Part model, mm, in its own coordinate system. A direction names the side the tool comes from. Round coordinates to 2 decimals unless told otherwise and drop trailing zeros. Loops run counter-clockwise (first coordinate to the right, second up) from the corner with the lowest first, then second, coordinate; pieces in that order, holes last. Notation, with made-up numbers: (37, -0.5) -> (77, -0.5) arc R24 ccw to (77, 11.5) -> close; hole circle Ø8 at (42.25, 15). An arc over 180 degrees is marked (long way). Answer as a JSON object with one key per item and string values. Group by question number.
from build123d import *

# Parameters (mm, degrees)
EXTRUDE_1_DEPTH             = 10.5
FILLET_1_R                  = 0.3
FILLET_2_R                  = 2
HOLE_WIZARD_M52_D           = 4.2
HOLE_WIZARD_M52_CSINK_D     = 5.05
HOLE_WIZARD_M52_CSINK_ANGLE = 90


with BuildPart() as part:
    # Эскиз1 → Бобышка-Вытянуть1 (new body, symmetric)
    with BuildSketch(Plane.XY):
        with BuildLine():
            Line((-4, 0), (4, 0))
            Line((4, 0), (4, -0.8))
            Line((4, -0.8), (6.5, -0.8))
            Line((6.5, -0.8), (6.5, -1.6))
            ThreePointArc((6.5, -1.6), (4.386776199, -4.87777644), (1.5, -7.5))
            Line((1.5, -7.5), (-1.5, -7.5))
            ThreePointArc((-1.5, -7.5), (-4.386776199, -4.87777644), (-6.5, -1.6))
            Line((-6.5, -1.6), (-6.5, -0.8))
            Line((-6.5, -0.8), (-4, -0.8))
            Line((-4, -0.8), (-4, 0))
        make_face()
    extrude(amount=EXTRUDE_1_DEPTH, both=True)

    # Скругление1
    fillet_1_edges = [part.edges().sort_by_distance(p)[0] for p in [
        (6.5, -0.8, 0),
        (6.5, -1.6, 0),
        (-6.5, -1.6, 0),
        (-6.5, -0.8, 0),
        (-4, 0, 0),
        (4, 0, 0),
    ]]
    fillet(fillet_1_edges, radius=FILLET_1_R)

    # Скругление2
    fillet_2_edges = [part.edges().sort_by_distance(p)[0] for p in [
        (1.5, -7.5, 0),
        (-1.5, -7.5, 0),
    ]]
    fillet(fillet_2_edges, radius=FILLET_2_R)

    # Отверстие обработанное метчиком M52 (through all)
    with Locations(Plane(origin=(0, 0, 0), x_dir=(1, 0, 0), z_dir=(0, 1, 0))):
        with Locations((0, -4.5)):
            CounterSinkHole(HOLE_WIZARD_M52_D / 2, HOLE_WIZARD_M52_CSINK_D / 2, counter_sink_angle=HOLE_WIZARD_M52_CSINK_ANGLE)

    # Эскиз5 → Повернуть1 (revolve)
    with BuildSketch(Plane(origin=(0, 0, 0), x_dir=(0, 0, -1), z_dir=(1, 0, 0))):
        with BuildLine():
            Line((6.5, -4.3), (6.5, -8.3))
            ThreePointArc((6.5, -8.3), (4.5, -6.3), (6.5, -4.3))
        make_face()
    revolve(axis=Axis((0, -4.3, -6.5), (0, -1, 0)))


solid = part.part
Item 1: Band-saw the part on B-B, the plane z = 4.5. List the corners of the cut face in (x, y) (3 decimals).
Item 2: Drill centre lines: line 1 (Z direction, x = 0, y = -2.5); line 2 (Y direction, x = -0.25, z = -1.5); line 3 (X direction, y = -7, z = 3). Where is each one in solid material? Low to high.
Item 3: Band-saw the part on D-D, the plane y = -5.5. List the corners of the cut face in (x, z).
Item 4: Two-plate mould, pull along Z, no slides. Class faces 5 (the face through (0.46, -4.01, 6.55)), 6 (the face through (0, -3, -10.5)), 7 (the face through (0, -3, 10.5)), 8 (the face through (1.5, -7.39, 8.28)): pulls with the +Z half, pulls with the -Z half, needs draft (parallel to the pull), parting line crosses it, or undercut.
Item 5: Band-saw the part on A-A, the plane x = 0. List the corners of the cut face in (y, z) (3 decimals).
Item 6: Drop flat-ended pins along their axis: pin 1 Ø1.8 at (x, z) = (-5, -1) entering from +Y; pin 2 Ø1.9 at (x, z) = (0.5, -9.5) entering from -Y; pin 3 Ø2 at (y, z) = (-5, 5.5) entering from -X. Give the stop position or say it passes through.
Item 7: Band-saw the part on C-C, the plane z = -3.25. List the corners of the cut face in (x, y).
Item 8: Which spindle directions (+Z, -Z, +X, -X, +Y, -Y) get a long thin tool onto all of the face, cutting with end or side? Do faces 1 (the face through (-5, -0.8, 0)), 2 (the face through (0, -7.5, 8)), 3 (the face through (1.5, -7.39, -3.29)), 4 (the face through (-1.5, -7.39, -3.29)). Say none if no direction does.
Entries:
{
 "1": {"outline": "(-6.5, -1.532) arc R0.3 ccw to (-6.471, -1.662) arc R15 ccw to (-2.1, -7.061) -> (-2.1, -0.425) -> (-2.525, 0) -> (-3.7, 0) arc R0.3 ccw to (-4, -0.3) -> (-4, -0.8) -> (-6.2, -0.8) arc R0.3 ccw to (-6.5, -1.1) -> close; (2.1, -7.061) arc R15 ccw to (6.471, -1.662) arc R0.3 ccw to (6.5, -1.532) -> (6.5, -1.1) arc R0.3 ccw to (6.2, -0.8) -> (4, -0.8) -> (4, -0.3) arc R0.3 ccw to (3.7, 0) -> (2.525, 0) -> (2.1, -0.425) -> close"},
 "2": {"line 1": "-10.5 to 2.4, 6.6 to 10.5", "line 2": "-7.5 to 0", "line 3": "-2.18 to -1.47, 1.47 to 2.18"},
 "3": {"outline": "(-3.83, -10.5) -> (3.83, -10.5) -> (3.83, 10.5) -> (-3.83, 10.5) -> close; hole circle Ø4.2 at (0, 4.5)"},
 "4": {"face 5": "undercut", "face 6": "pulls with the -Z half", "face 7": "pulls with the +Z half", "face 8": "needs draft"},
 "5": {"outline": "(-7.5, -10.5) -> (0, -10.5) -> (0, 1.975) -> (-0.425, 2.4) -> (-7.5, 2.4) -> (-7.5, -4.9) arc R2 ccw to (-7.5, -8.1) -> close; (-7.5, 6.6) -> (-0.425, 6.6) -> (0, 7.025) -> (0, 10.5) -> (-7.5, 10.5) -> close"},
 "6": {"pin 1": "y = -0.8", "pin 2": "y = -7.5", "pin 3": "x = -5.08"},
 "7": {"outline": "(-6.5, -1.53) arc R0.3 ccw to (-6.47, -1.66) arc R15 ccw to (-2.07, -7.09) arc R2 ccw to (-0.85, -7.5) -> (0.85, -7.5) arc R2 ccw to (2.07, -7.09) arc R15 ccw to (6.47, -1.66) arc R0.3 ccw to (6.5, -1.53) -> (6.5, -1.1) arc R0.3 ccw to (6.2, -0.8) -> (4, -0.8) -> (4, -0.3) arc R0.3 ccw to (3.7, 0) -> (-3.7, 0) arc R0.3 ccw to (-4, -0.3) -> (-4, -0.8) -> (-6.2, -0.8) arc R0.3 ccw to (-6.5, -1.1) -> close"},
 "8": {"face 1": "+Z, -Z, -X, +Y", "face 2": "+Z, +X, -X, -Y", "face 3": "+X, -Y", "face 4": "-X, -Y"}
}
